Build history of the part. All positions in model axes, mm. Face numbers are marked on the shaded views. Coordinates: 2 decimals unless noted, no trailing zeros. Order: outer loops, then holes, each group sorted by start corner. A loop starts at its lowest first (then second) coordinate and runs counter-clockwise, first axis right, second up. Notation, with made-up numbers: (-4.75, 86.5) - (17.25, 86.5) arc R23 ccw to (17.25, 120.5) - close; hole circle Ø11 at (-13, -33). An arc over 180 degrees is marked (long way). One line per item, written item: value.
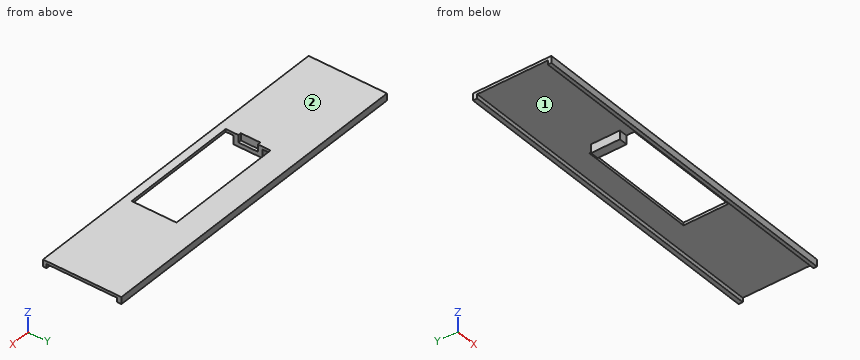
from build123d import *

# Parameters (mm, degrees)
F0_W      = 240
F0_H      = 56
F0_W_2    = 85
F0_H_2    = 32
F1_DEPTH  = 2
F2_W      = 2.2
F2_H      = 14
F3_DEPTH  = 25
F5_DEPTH  = 3.2
F6_W      = 2.2
F6_H      = 14
F7_DEPTH  = 3
F8_W      = 240
F8_H      = 3
F9_DEPTH  = 3
F8_H_2    = 2.5
F10_DEPTH = 3


with BuildPart() as f1:
    # F0 (on Top) → F1 (new body)
    with BuildSketch(Plane.XY):
        with Locations((13.640271, 28)):
            Rectangle(F0_W, F0_H)
        with Locations((17.96643, 21.5)):
            Rectangle(F0_W_2, F0_H_2, mode=Mode.SUBTRACT)
    extrude(amount=F1_DEPTH)

    # F2 (on face) → F3 (cut)
    with BuildSketch(Plane.XY.offset(2)):
        with Locations((-25.63357, 21.5)):
            Rectangle(F2_W, F2_H)
    extrude(amount=-F3_DEPTH, mode=Mode.SUBTRACT)

    # F4 (on face) → F5 (join)
    with BuildSketch(Plane(origin=(0, 0, 0), x_dir=(1, 0, 0), z_dir=(0, 0, -1))):
        Polygon((-24.53357, -14.5), (-24.53357, -11.051576), (-30.502366, -11.051576), (-30.502366, -31.678651), (-24.53357, -31.678651), (-24.53357, -28.5), (-26.73357, -28.5), (-26.73357, -14.5), align=None)
    extrude(amount=F5_DEPTH)

    # F6 (on face) → F7 (join)
    with BuildSketch(Plane(origin=(0, 0, -3.2), x_dir=(1, 0, 0), z_dir=(0, 0, -1))):
        Polygon((-24.53357, -14.5), (-24.53357, -11.051576), (-30.502366, -11.051576), (-30.502366, -31.678651), (-24.53357, -31.678651), (-24.53357, -28.5), (-26.73357, -28.5), (-26.73357, -14.5), align=None)
        with Locations((-25.63357, -21.5)):
            Rectangle(F6_W, F6_H)
    extrude(amount=F7_DEPTH)

    # F8 (on face) → F9 (join)
    with BuildSketch(Plane(origin=(0, 0, 0), x_dir=(1, 0, 0), z_dir=(0, 0, -1))):
        with Locations((13.640271, -54.5)):
            Rectangle(F8_W, F8_H)
    extrude(amount=F9_DEPTH)

    # F8 (on face) → F10 (join)
    with BuildSketch(Plane(origin=(0, 0, 0), x_dir=(1, 0, 0), z_dir=(0, 0, -1))):
        with Locations((13.640271, -1.25)):
            Rectangle(F8_W, F8_H_2)
    extrude(amount=F10_DEPTH)


solid = f1.part
1. Band-saw the part on C-C, the plane x = 68. Give the cut face in (y, z).
Values found:
outline: (0, -3) - (2.5, -3) - (2.5, 0) - (53, 0) - (53, -3) - (56, -3) - (56, 2) - (0, 2) - close
2. Band-saw the part on B-B, the plane y = 18.5. Give the cut face in (x, z), and give its area (3 significant figures).
Values found:
outline: (-106.36, 0) - (-30.5, 0) - (-30.5, -6.2) - (-24.53, -6.2) - (-24.53, -3.2) - (-26.73, -3.2) - (-26.73, 2) - (-106.36, 2) - close; (60.47, 0) - (133.64, 0) - (133.64, 2) - (60.47, 2) - close
area: 336 mm2
3. Flat gauge pins, fed straight in: P1, Ø2, axis at x = -34.5, y = 1, coming from the -Z side; P2, Ø6, axis at x = 19.5, y = 7.5, coming from the -Z side; P3, Ø1.8, axis at x = -27, z = -4, coming from the -Y side. Where does each tip first touch, or does it go through?
Values found:
P1: stops at z = -3
P2: stops at z = 0
P3: stops at y = 11.05
4. Two-plate mould, pull along Y, no slides. Class the marked faces 1 and 2: pulls with the +Y half, pulls with the -Y half, needs draft (parallel to the pull), parting line crosses it, or undercut.
Values found:
face 1: undercut
face 2: needs draft
5. Probe line 1 along X through (y, z) = (17.5, 0.25); line 2 along Y through (x, z) = (-46, -2); line 3 along X through (y, z) = (11, 1). List the from-to ranges inside material, lowest first.
Values found:
line 1: x = -106.36 to -26.73, 60.47 to 133.64
line 2: y = 0 to 2.5, 53 to 56
line 3: x = -106.36 to -24.53, 60.47 to 133.64
6. Band-saw the part on A-A, the plane x = 34. Give the cut face in (y, z).
Values found:
outline: (0, -3) - (2.5, -3) - (2.5, 0) - (5.5, 0) - (5.5, 2) - (0, 2) - close; (37.5, 0) - (53, 0) - (53, -3) - (56, -3) - (56, 2) - (37.5, 2) - close
7. Band-saw the part on D-D, the plane y = 46.5. Give the cut face in (x, z).
Values found:
outline: (-106.36, 0) - (133.64, 0) - (133.64, 2) - (-106.36, 2) - close
